```python
from build123d import *

# Parameters (mm, degrees)
F0_W     = 700
F0_H     = 1300
F0_W_2   = 600
F0_H_2   = 741.365468
F0_W_3   = 275
F0_H_3   = 411.491126
F0_H_4   = 409.27878
F1_DEPTH = 40
F2_SIZE  = 10


with BuildPart() as f1:
    # F0 (on Top) → F1 (new body)
    with BuildSketch(Plane.XY):
        with Locations((-1.148704, 142.788631)):
            Rectangle(F0_W, F0_H)
        with Locations((-1.148704, -86.528635)):
            Rectangle(F0_W_2, F0_H_2, mode=Mode.SUBTRACT)
        with Locations((-163.648704, 539.899662)):
            Rectangle(F0_W_3, F0_H_3, mode=Mode.SUBTRACT)
        with Locations((161.351296, 538.793489)):
            Rectangle(F0_W_3, F0_H_4, mode=Mode.SUBTRACT)
    extrude(amount=F1_DEPTH)

    # F2
    f2_edges = [f1.edges().sort_by_distance(p)[0] for p in [
        (-1.148704, -457.211369, 40),
        (298.851296, -86.528635, 40),
        (-1.148704, 284.154099, 40),
        (-301.148704, -86.528635, 40),
        (23.851296, 538.793489, 40),
        (161.351296, 334.154099, 40),
        (-163.648704, 334.154099, 40),
        (-26.148704, 539.899662, 40),
        (298.851296, 538.793489, 40),
        (-301.148704, 539.899662, 40),
        (-163.648704, 745.645225, 40),
        (161.351296, 743.432879, 40),
    ]]
    chamfer(f2_edges, length=F2_SIZE)


solid = f1.part
```
CAD build for the part. Positions are in the model's coordinates, mm. A direction names the side the tool comes from. Coordinates: 2 decimals unless noted, no trailing zeros. Write each loop counter-clockwise with the first axis right and the second up, starting at its lowest first coordinate (ties: lowest second). Pieces come first, ordered by that corner, then holes.
(1) Cut at C-C, the plane z = 8. List the corners of the cut face in (x, y), and give its area (3 significant figures).
(2) Cut at D-D, the plane y = -282. List the corners of the cut face in (x, z), and give its area (3 significant figures).
(3) Cut at A-A, the plane y = 591. List the corners of the cut face in (x, z).
(4) 3-axis set-ups, long thin cutter, end or side, ignore diameter. For faces 1 (the face through (-351.149, 134, 20)), 2 (the face through (-166, 745.645, 15)): which of +Z, -Z, +X, -X, +Y, -Y reach the whole face in a straight line?
(5) Two-plate mould, pull along Y, no slides. Class faces 3 (the face through (-3, 387, 40)), 4 (the face through (-6, -507.211, 20)), 5 (the face through (298.851, 536, 15)), 6 (the face through (-6, 792.789, 20)): +Y half, -Y half, draft (parallel to the pull), parting line (faces both ways), or undercut.
(6) Drill centre lines: probe 1 along X at (y, z) = (439.5, 29.5); probe 2 along Y at (x, z) = (289, 4); probe 3 along Y at (x, z) = (-158, 6). Where is each one in solid material? Low to high.
(7) Cut at B-B, the plane x = 125. List the corners of the cut face in (y, z), and give its area (3 significant figures).
Geometry says:
1. outline: (-351.15, -507.21) - (348.85, -507.21) - (348.85, 792.79) - (-351.15, 792.79) - close; hole (-301.15, -457.21) - (298.85, -457.21) - (298.85, 284.15) - (-301.15, 284.15) - close; hole (-301.15, 334.15) - (-26.15, 334.15) - (-26.15, 745.65) - (-301.15, 745.65) - close; hole (23.85, 334.15) - (298.85, 334.15) - (298.85, 743.43) - (23.85, 743.43) - close
1. area: 239,000 mm2
2. outline: (-351.15, 0) - (-301.15, 0) - (-301.15, 30) - (-311.15, 40) - (-351.15, 40) - close; (298.85, 0) - (348.85, 0) - (348.85, 40) - (308.85, 40) - (298.85, 30) - close
2. area: 3,900 mm2
3. outline: (-351.15, 0) - (-301.15, 0) - (-301.15, 30) - (-311.15, 40) - (-351.15, 40) - close; (-26.15, 0) - (23.85, 0) - (23.85, 30) - (13.85, 40) - (-16.15, 40) - (-26.15, 30) - close; (298.85, 0) - (348.85, 0) - (348.85, 40) - (308.85, 40) - (298.85, 30) - close
4. face 1: +Z, -Z, -X, +Y, -Y
4. face 2: +Z, -Z
5. face 3: draft
5. face 4: -Y half
5. face 5: undercut
5. face 6: +Y half
6. probe 1: x = -351.15 to -301.15, -26.15 to 23.85, 298.85 to 348.85
6. probe 2: y = -507.21 to -457.21, 284.15 to 334.15, 743.43 to 792.79
6. probe 3: y = -507.21 to -457.21, 284.15 to 334.15, 745.65 to 792.79
7. outline: (-507.21, 0) - (-457.21, 0) - (-457.21, 30) - (-467.21, 40) - (-507.21, 40) - close; (284.15, 0) - (334.15, 0) - (334.15, 30) - (324.15, 40) - (294.15, 40) - (284.15, 30) - close; (743.43, 0) - (792.79, 0) - (792.79, 40) - (753.43, 40) - (743.43, 30) - close
7. area: 5,770 mm2
